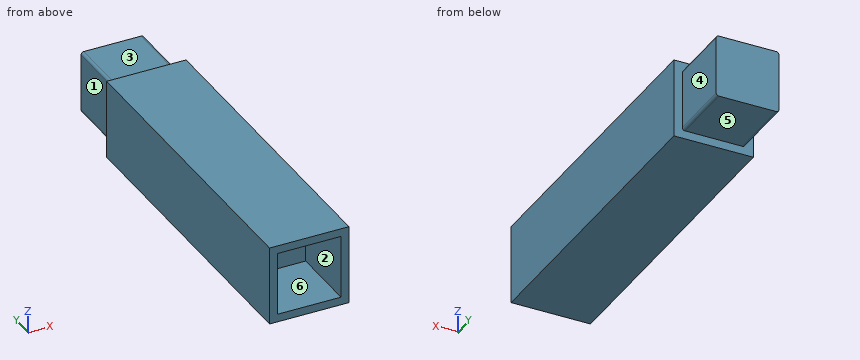
```python
from build123d import *

# Parameters (mm, degrees)
SKETCH1_W           = 30
SKETCH1_H           = 30
BOSS_EXTRUDE1_DEPTH = 120
SKETCH2_W           = 23.7
SKETCH2_H           = 23.7
BOSS_EXTRUDE2_DEPTH = 25
SKETCH3_W           = 24
SKETCH3_H           = 24
CUT_EXTRUDE1_DEPTH  = 26
FILLET1_R           = 1


with BuildPart() as part:
    # Sketch1 → Boss-Extrude1 (new body)
    with BuildSketch(Plane(origin=(0, 0, 0), x_dir=(1, 0, 0), z_dir=(0, 1, 0))):
        Rectangle(SKETCH1_W, SKETCH1_H)
    extrude(amount=BOSS_EXTRUDE1_DEPTH)

    # Sketch2 → Boss-Extrude2 (add)
    with BuildSketch(Plane(origin=(0, 120, 0), x_dir=(1, 0, 0), z_dir=(0, 1, 0))):
        Rectangle(SKETCH2_W, SKETCH2_H)
    extrude(amount=BOSS_EXTRUDE2_DEPTH)

    # Sketch3 → Cut-Extrude1 (cut)
    with BuildSketch(Plane.XZ):
        Rectangle(SKETCH3_W, SKETCH3_H)
    extrude(amount=-CUT_EXTRUDE1_DEPTH, mode=Mode.SUBTRACT)

    # Fillet1
    fillet1_edges = [part.edges().sort_by_distance(p)[0] for p in [
        (11.85, 132.5, 11.85),
        (11.85, 132.5, -11.85),
        (-11.85, 132.5, -11.85),
        (-11.85, 132.5, 11.85),
    ]]
    fillet(fillet1_edges, radius=FILLET1_R)


solid = part.part
```
Part model, mm, in its own coordinate system. Face numbers are marked on the shaded views. A direction names the side the tool comes from. Round coordinates to 2 decimals unless told otherwise and drop trailing zeros. Write each loop counter-clockwise with the first axis right and the second up, starting at its lowest first coordinate (ties: lowest second). Pieces come first, ordered by that corner, then holes. Notation, with made-up numbers: (79, -4) -> (123, -4) arc R21 ccw to (123, 25) -> close; hole circle Ø3 at (60, 67). An arc over 180 degrees is marked (long way). Return JSON: item names as keys, results as strings. Group by question number.
Q1. Saw through at B-B on x = 9.25. Write the cut outline in (y, z).
Q2. Mould opens along X. For the marked faces 1, 2 and 3 say: pulls with the +X half, pulls with the -X half, needs draft (parallel to the pull), parting line crosses it, or undercut.
Q3. Saw through at A-A on y = 24.5. Write the cut outline in (x, z).
Q4. Pin check, flat tips, straight feed: pin 1 (6.5 mm diameter, centred on x = 1.5, y = 129.5, fed in from +Z); pin 2 (12 mm diameter, centred on x = -10, z = -7.5, fed in from -Y); pin 3 (17.5 mm diameter, centred on x = 1.5, y = 132.5, fed in from -Z); pin 4 (7 mm diameter, centred on x = 5, z = 1, fed in from -Y). Stop position of each tip, or through.
Q5. Probe L1, parallel to Z at x = 11.75, y = 10; L2, parallel to Y at x = 3.5, z = -3; L3, parallel to X at y = 125, z = 2.75. List the from-to ranges inside material, lowest first. Write a range as [from, to].
Q6. Which spindle directions (+Z, -Z, +X, -X, +Y, -Y) get a long thin tool onto all of the face, cutting with end or side? Do the marked faces 4, 5 and 6. Say none if no direction does.
Q7. Saw through at C-C on z = 2.25. Write the cut outline in (x, y).
Answer:
{
 "1": {"outline": "(0, -15) -> (120, -15) -> (120, -11.85) -> (145, -11.85) -> (145, 11.85) -> (120, 11.85) -> (120, 15) -> (0, 15) -> (0, 12) -> (26, 12) -> (26, -12) -> (0, -12) -> close"},
 "2": {"face 1": "pulls with the -X half", "face 2": "undercut", "face 3": "needs draft"},
 "3": {"outline": "(-15, -15) -> (15, -15) -> (15, 15) -> (-15, 15) -> close; hole (-12, -12) -> (12, -12) -> (12, 12) -> (-12, 12) -> close"},
 "4": {"pin 1": "z = 11.85", "pin 2": "y = 0", "pin 3": "z = -11.85", "pin 4": "y = 26"},
 "5": {"L1": "[-15, -12], [12, 15]", "L2": "[26, 145]", "L3": "[-11.85, 11.85]"},
 "6": {"face 4": "+Z, -Z, +X, +Y", "face 5": "-Z, +X, -X, +Y", "face 6": "-Y"},
 "7": {"outline": "(-15, 0) -> (-12, 0) -> (-12, 26) -> (12, 26) -> (12, 0) -> (15, 0) -> (15, 120) -> (11.85, 120) -> (11.85, 145) -> (-11.85, 145) -> (-11.85, 120) -> (-15, 120) -> close"}
}
